Autodesk Inventor part; units mm, degrees
ref_plane "YZ Plane" through (0, 0, 0) normal (1, 0, 0) x (0, 1, 0)
ref_plane "XZ Plane" through (0, 0, 0) normal (0, 1, 0) x (-1, 0, 0)
ref_plane "XY Plane" through (0, 0, 0) normal (0, 0, 1) x (1, 0, 0)
sketch "Sketch1" plane through (0, 0, 0) normal (1, 0, 0) x (0, 1, 0)
  line L0 (3.175, 0) -> (240.665, 0)
  line L1 (243.84, -3.175) -> (243.84, -6.985)
  line L2 (240.665, -10.16) -> (3.175, -10.16)
  line L3 (0, -6.985) -> (0, -3.175)
  arc A0 (243.84, -3.175) -> (240.665, 0) centre (240.665, -3.175) ccw
  arc A1 (240.665, -10.16) -> (243.84, -6.985) centre (240.665, -6.985) ccw
  arc A2 (3.175, 0) -> (0, -3.175) centre (3.175, -3.175) ccw
  arc A3 (0, -6.985) -> (3.175, -10.16) centre (3.175, -6.985) ccw
  line L4 (0, -5.08) -> (243.84, -5.08) construction
  point P0 (0, 0)
  point P1 (243.84, -10.16)
  point P2 (243.84, 0)
  point P3 (0, -10.16)
  point P4 (20.32, -5.08)
  point P5 (60.96, -5.08)
  point P6 (101.6, -5.08)
  point P7 (142.24, -5.08)
  point P8 (182.88, -5.08)
  point P9 (223.52, -5.08)
  dimension "d0" = 243.84
  dimension "d1" = 10.16
  dimension "d2" = 3.175
  dimension "d3" = 20.32
  dimension "d6" = 40.64
  dimension "d21" = 101.6
extrude "Extrusion1" add sketch "Sketch1" along normal blind 2.794
hole "Hole3" at (0, 20.32, -5.08) at (0, 60.96, -5.08) at (0, 101.6, -5.08) at (0, 142.24, -5.08) at (0, 182.88, -5.08) at (0, 223.52, -5.08) direction (1, 0, 0) diameter 4 end through all
properties part number "ArmSpacer6" material "Polycarbonate, Smoke"
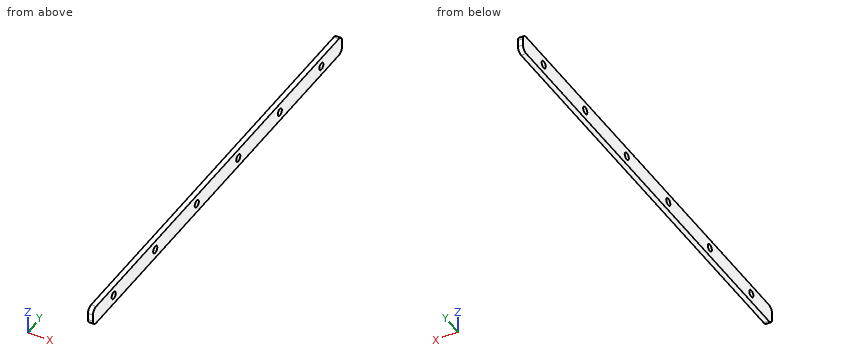
Can you work these out from the model? Positions are in its coordinate system, mm. Coordinates: 2 decimals unless noted, no trailing zeros. Order: outer loops, then holes, each group sorted by start corner. A loop starts at its lowest first (then second) coordinate and runs counter-clockwise, first axis right, second up. Notation, with made-up numbers: (-23, -24.5) - (15, -24.5) arc R12 ccw to (15, -11.5) - close; hole circle Ø4 at (43, 29). An arc over 180 degrees is marked (long way). Answer as a JSON object with one key per item and string values. Group by question number.
Q1. Imagine slicing it at B-B (y = 223.52). Please give me the cut outline in (x, z).
Q2. Imagine slicing it at C-C (x = 0.5). Please give me the cut outline in (y, z) (3 decimals), and give its area (3 significant figures).
Q3. I need wall thicknesses on line 1 (Z direction, x = 2.05, y = 142.24); line 2 (Y direction, x = 0.15, z = -2.75); line 3 (Z direction, x = 1.5, y = 62). Which ranges of each line are inside material? Lowest first, please. Write a range as from..to.
Q4. Imagine slicing it at A-A (z = -5.08). Please give me the cut outline in (x, y), and give its area (3 significant figures).
Determined:
{
 "1": {"outline": "(0, -10.16) - (2.79, -10.16) - (2.79, -7.08) - (0, -7.08) - close; (0, -3.08) - (2.79, -3.08) - (2.79, 0) - (0, 0) - close"},
 "2": {"outline": "(0, -6.985) arc R3.175 ccw to (3.175, -10.16) - (240.665, -10.16) arc R3.175 ccw to (243.84, -6.985) - (243.84, -3.175) arc R3.175 ccw to (240.665, 0) - (3.175, 0) arc R3.175 ccw to (0, -3.175) - close; hole circle Ø4 at (20.32, -5.08); hole circle Ø4 at (60.96, -5.08); hole circle Ø4 at (101.6, -5.08); hole circle Ø4 at (142.24, -5.08); hole circle Ø4 at (182.88, -5.08); hole circle Ø4 at (223.52, -5.08)", "area": "2,390 mm2"},
 "3": {"line 1": "z = -10.16..-7.08, -3.08..0", "line 2": "y = 0.03..243.81", "line 3": "z = -10.16..-6.79, -3.37..0"},
 "4": {"outline": "(0, 0) - (2.79, 0) - (2.79, 18.32) - (0, 18.32) - close; (0, 22.32) - (2.79, 22.32) - (2.79, 58.96) - (0, 58.96) - close; (0, 62.96) - (2.79, 62.96) - (2.79, 99.6) - (0, 99.6) - close; (0, 103.6) - (2.79, 103.6) - (2.79, 140.24) - (0, 140.24) - close; (0, 144.24) - (2.79, 144.24) - (2.79, 180.88) - (0, 180.88) - close; (0, 184.88) - (2.79, 184.88) - (2.79, 221.52) - (0, 221.52) - close; (0, 225.52) - (2.79, 225.52) - (2.79, 243.84) - (0, 243.84) - close", "area": "614 mm2"}
}
